Work out the finished part from the listing and answer in its coordinate system (mm). Round coordinates to 2 decimals unless told otherwise and drop trailing zeros. Write each loop counter-clockwise with the first axis right and the second up, starting at its lowest first coordinate (ties: lowest second). Pieces come first, ordered by that corner, then holes.
from build123d import *

# Parameters (mm, degrees)
EXTRUDE_1_DEPTH = 5.65
FILLET_1_R      = 0.5
OTHER_START     = -9.109345257
OTHER_1_DEPTH   = 18.218690514
OTHER_1_2_DEPTH = 0.442344722
OTHER_START_2   = 8.668200897
OTHER_1_3_DEPTH = 0.44114436


# Read off the part's stored shape, not the designer's step: 型腔1
with BuildPart() as part:
    # 草图1 → 凸台-拉伸1 (new body)
    with BuildSketch(Plane.XY):
        with BuildLine():
            Line((-9.3, 0), (-9.3, -15.9))
            Line((-9.3, -15.9), (9.3, -15.9))
            Line((9.3, -15.9), (9.3, 0))
            ThreePointArc((9.3, 0), (0, 9.3), (-9.3, 0))
        make_face()
    extrude(amount=EXTRUDE_1_DEPTH)

    # 圆角1
    fillet_1_edges = [part.edges().sort_by_distance(p)[0] for p in [
        (9.3, -15.9, 2.825),
        (-9.3, -15.9, 2.825),
    ]]
    fillet(fillet_1_edges, radius=FILLET_1_R)

    # 型腔1 outline → 型腔1 (cut)
    with BuildSketch(Plane.YZ.offset(OTHER_START)):
        Polygon((-15.873817403, 5.640486893), (-15.792817403, 5.640486893), (-15.792817403, 5.65), (-15.9, 5.65), (-15.9, 5.521595656), (-15.873817403, 5.54823926), align=None)
    extrude(amount=OTHER_1_DEPTH, mode=Mode.SUBTRACT)

    # Other 1 2 outline → Other 1 2 (cut)
    with BuildSketch(Plane.YZ.offset(OTHER_START)):
        Polygon((-15.873817403, 5.54823926), (-15.792817403, 5.63066546), (-15.792817403, 5.640486893), (-15.873817403, 5.640486893), align=None)
    extrude(amount=OTHER_1_2_DEPTH, mode=Mode.SUBTRACT)

    # Other 1 3 outline → Other 1 3 (cut)
    with BuildSketch(Plane.YZ.offset(OTHER_START_2)):
        Polygon((-15.873817403, 5.54823926), (-15.792817403, 5.63066546), (-15.792817403, 5.640486893), (-15.873817403, 5.640486893), align=None)
    extrude(amount=OTHER_1_3_DEPTH, mode=Mode.SUBTRACT)


solid = part.part
Q1. Given pin 1 (10 mm diameter, centred on x = 2.5, y = 5, fed in from -Z), flat-ended and moving along its own axis, determine where the tip first touches the part or whether it passes through.
Q2. Find section A-A (z = 5.2). Determine the outline of the cut face in (x, y).
Q3. Find the intervals of material crossed by L1, parallel to Y at x = -4.5, z = 0.3; L2, parallel to Y at x = 0.5, z = 1.65; L3, parallel to X at y = 1, z = 1.45, in increasing order.
Q4. Find section C-C (y = 2.75). Determine the outline of the cut face in (x, z), plus the area to 3 significant figures.
Q5. Find section B-B (y = 6.5). Determine the outline of the cut face in (x, z), plus the area to 3 significant figures.
Report:
1. pin 1: stops at z = 0
2. outline: (-9.3, -15.4) arc R0.5 ccw to (-8.8, -15.9) - (8.8, -15.9) arc R0.5 ccw to (9.3, -15.4) - (9.3, 0) arc R9.3 ccw to (-9.3, 0) - close
3. L1: y = -15.9 to 8.14
3. L2: y = -15.9 to 9.29
3. L3: x = -9.25 to 9.25
4. outline: (-8.88, 0) - (8.88, 0) - (8.88, 5.65) - (-8.88, 5.65) - close
4. area: 100 mm2
5. outline: (-6.65, 0) - (6.65, 0) - (6.65, 5.65) - (-6.65, 5.65) - close
5. area: 75.2 mm2
